```python
from build123d import *

# Parameters (mm, degrees)
SKETCH1_W           = 2
SKETCH1_H           = 22
REVOLVE1_ANGLE      = 30
BOSS_EXTRUDE2_DEPTH = 57
CUT_EXTRUDE1_START  = -6.211657082
CUT_EXTRUDE1_DEPTH  = 12.423314164
SKETCH16_W          = 8
SKETCH16_H          = 8
REVOLVE2_ANGLE      = 1
FILLET2_R           = 3


# Read off the part's stored shape, not the designer's step: Cut-Extrude1
with BuildPart() as part:
    # Sketch1 → Revolve1 (revolve, symmetric)
    with BuildSketch(Plane.XY) as revolve1_sk:
        with Locations((100, 5)):
            Rectangle(SKETCH1_W, SKETCH1_H)
    revolve(axis=Axis((0, 12.85, 0), (0, -1, 0)), revolution_arc=REVOLVE1_ANGLE / 2)
    revolve(revolve1_sk.sketch, axis=Axis((0, 12.85, 0), (0, 1, 0)), revolution_arc=REVOLVE1_ANGLE / 2)

    # Sketch13 → Boss-Extrude2 (add, along a direction that is not the sketch's normal)
    with BuildSketch(Plane(origin=(0, 0, 0), x_dir=(0.9659258262890682, 0, 0.25881904510252124), z_dir=(-0.25881904510252124, 0, 0.9659258262890682))):
        Polygon((80.681483474, -4.141104722), (119.318516526, 6.211657082), (119.318516526, 4.141104722), (80.681483474, -6.211657082), align=None)
    extrude(amount=-BOSS_EXTRUDE2_DEPTH, dir=(0, 0, 1))

    # Cut-Extrude1 outline → Cut-Extrude1 (cut)
    with BuildSketch(Plane(origin=(0, 0, 0), x_dir=(1, 0, 0), z_dir=(0, 1, 0)).offset(CUT_EXTRUDE1_START)):
        with BuildLine():
            Line((91.762953497, 24.587809285), (101.42221176, 27.175999736))
            ThreePointArc((101.42221176, 27.175999736), (105, 0), (101.42221176, -27.175999736))
            Line((101.42221176, -27.175999736), (115.252836667, -30.88190451))
            Line((115.252836667, -30.88190451), (115.252836667, 26.11809549))
            Line((115.252836667, 26.11809549), (77.932328591, 36.11809549))
            Line((77.932328591, 36.11809549), (77.932328591, -20.88190451))
            Line((77.932328591, -20.88190451), (91.762953497, -24.587809285))
            ThreePointArc((91.762953497, -24.587809285), (95, 0), (91.762953497, 24.587809285))
        make_face()
    extrude(amount=CUT_EXTRUDE1_DEPTH, mode=Mode.SUBTRACT)

    # Sketch16 → Revolve2 (revolve, symmetric)
    with BuildSketch(Plane.XY) as revolve2_sk:
        with Locations((100, -10)):
            Rectangle(SKETCH16_W, SKETCH16_H)
    revolve(axis=Axis((0, 12.85, 0), (0, -1, 0)), revolution_arc=REVOLVE2_ANGLE / 2)
    revolve(revolve2_sk.sketch, axis=Axis((0, 12.85, 0), (0, 1, 0)), revolution_arc=REVOLVE2_ANGLE / 2)

    # Fillet2
    fillet2_edges = [part.edges().sort_by_distance(p)[0] for p in [
        (99, -6, 0),
        (101, -6, 0),
    ]]
    fillet(fillet2_edges, radius=FILLET2_R - 0.0001)  # a hair under: the kernel refuses the full size


solid = part.part
```
Input: part model. Units: mm. Frame: model coordinates. A direction names the side the tool comes from. Coordinates: 2 decimals unless noted, no trailing zeros. Write each loop counter-clockwise with the first axis right and the second up, starting at its lowest first coordinate (ties: lowest second). Pieces come first, ordered by that corner, then holes. Notation, with made-up numbers: (-29, 44.25) - (17, 44.25) arc R14 cw to (17, 59.25) - close; hole circle Ø3 at (23.5, -9). An arc over 180 degrees is marked (long way). Put each result on its own line as item: value. Start each with the question number.
1) Reachability of faces 1 (the face through (96.72, 1.07, 0.41)), 2 (the face through (95, -1, 0)), 3 (the face through (101.459, 2.385, 0.137)) from +Z, -Z, +X, -X, +Y, -Y: full face, straight path, thin tool, end or side. Return the list, or none.
2) Mould query, pull axis X, two halves, no side actions, for faces 4 (the face through (96.62, 3.42, 25.89)), 5 (the face through (95.657, -1.295, 0.128)), 6 (the face through (100, -14, 0)), 7 (the face through (99, -2, 0)). Classes: pulls with the +X half, pulls with the -X half, needs draft (parallel to the pull), parting line crosses it, or undercut.
3) Cut plane D-D (z = 13). Return the cut outline in (x, y), plus the area to 3 significant figures.
4) Cut plane C-C (y = 9). Return the cut outline in (x, z).
5) Cut plane B-B (z = 21). Return the cut outline in (x, y).
6) Ray query, L1, parallel to X at y = -6.5, z = 0; L2, parallel to Y at x = 98, z = -17; L3, parallel to Z at x = 98.25, y = -8. Return the intervals inside material, ascending.
7) Cut plane A-A (x = 93). Return the cut outline in (y, z), plus the area to 3 significant figures.
8) Contact query for flat-ended pins moving along their axis: pin 1 (1 mm diameter, centred on x = 97, z = 9.5, fed in from -Y); pin 2 (1.5 mm diameter, centred on x = 98, z = -13.5, fed in from -Y); pin 3 (2 mm diameter, centred on x = 102, y = 1, fed in from +Z); pin 4 (2 mm diameter, centred on y = 7.5, z = -6, fed in from -X). Output: stop coordinate, or through.
Resolved:
1. face 1: -X, +Y
1. face 2: -X, +Y, -Y
1. face 3: +Y
2. face 4: pulls with the -X half
2. face 5: undercut
2. face 6: needs draft
2. face 7: undercut
3. outline: (94.11, -1.72) - (98.14, -0.61) - (98.14, -6) - (100.16, -6) - (100.16, -0.05) - (104.19, 1.07) - (104.19, 3.14) - (100.16, 2.02) - (100.16, 16) - (98.14, 16) - (98.14, 1.47) - (94.11, 0.35) - close
3. area: 61.1 mm2
4. outline: (95.63, -25.62) - (97.56, -26.14) arc R101 ccw to (97.56, 26.14) - (95.63, 25.62) arc R99 cw to start
5. outline: (92.65, -2.13) - (96.75, -0.99) - (96.75, -6) - (98.79, -6) - (98.79, -0.42) - (102.88, 0.71) - (102.88, 2.78) - (98.79, 1.65) - (98.79, 16) - (96.75, 16) - (96.75, 1.08) - (92.65, -0.06) - close
6. L1: x = 96 to 104
6. L2: y = -6 to 16
6. L3: z = -0.86 to 0.86
7. outline: (-2.03, -24.92) - (0.04, -24.92) - (0.04, -19.39) - (-2.03, -19.39) - close; (-2.03, 19.39) - (0.04, 19.39) - (0.04, 24.92) - (-2.03, 24.92) - close
7. area: 22.9 mm2
8. pin 1: stops at y = -1.06
8. pin 2: stops at y = -6
8. pin 3: stops at z = 27.18
8. pin 4: stops at x = 98.75
